Source: CAD feature listing. Evaluate the final solid. Frame: model axes, mm. A direction names the side the tool comes from. Coordinates: 2 decimals unless noted, no trailing zeros. Order: outer loops, then holes, each group sorted by start corner. A loop starts at its lowest first (then second) coordinate and runs counter-clockwise, first axis right, second up.
```python
from build123d import *

# Parameters (mm, degrees)
F0_W     = 46.8558967113
F0_H     = 64.1569495201
F1_DEPTH = 127
F2_R     = 23.3551916442
F2_W     = 46.8558967113
F2_H     = 64.1569495201
F2_R_2   = 20.2511661355
F3_DEPTH = 25.4


# Not quite as in the source:
# - a feature of the source that left no trace in its solid (it failed there, or was rolled back) is left out


with BuildPart() as f1:
    # F0 (on Top) → F1 (new body)
    with BuildSketch(Plane.XY):
        Rectangle(F0_W, F0_H)
    extrude(amount=F1_DEPTH)

    # F0 (on Top) + F2 (on face) → F3 (join)
    with BuildSketch(Plane.XY):
        Rectangle(F0_W, F0_H)
    with BuildSketch(Plane.XY):
        with BuildLine():
            Line((33.4399625558, -78.6570606891), (35.4419024774, -78.6570606891))
            Line((35.4419024774, -78.6570606891), (35.4419024774, 78.6570606891))
            ThreePointArc((35.4419024774, 78.6570606891), (0, 114.0989631665), (-35.4419024774, 78.6570606891))
            Line((-35.4419024774, 78.6570606891), (-35.4419024774, -78.6570606891))
            Line((-35.4419024774, -78.6570606891), (-33.4399625558, -78.6570606891))
            ThreePointArc((-33.4399625558, -78.6570606891), (0, -112.0970232449), (33.4399625558, -78.6570606891))
        make_face()
        with Locations((0, -78.6570606891)):
            Circle(F2_R, mode=Mode.SUBTRACT)
        Rectangle(F2_W, F2_H, mode=Mode.SUBTRACT)
        with Locations((0, 78.6570606891)):
            Circle(F2_R_2, mode=Mode.SUBTRACT)
    extrude(amount=F3_DEPTH)


solid = f1.part
```
1. Section query A-A on x = 0. Return loops of the section in (y, z), plus the area to 3 significant figures.
Findings:
outline: (-112.1, 0) - (-102.01, 0) - (-102.01, 25.4) - (-112.1, 25.4) - close; (-55.3, 0) - (58.41, 0) - (58.41, 25.4) - (32.08, 25.4) - (32.08, 127) - (-32.08, 127) - (-32.08, 25.4) - (-55.3, 25.4) - close; (98.91, 0) - (114.1, 0) - (114.1, 25.4) - (98.91, 25.4) - close
area: 10,000 mm2
2. Ray query, line 1 (Y direction, x = 0, z = 12); line 2 (Z direction, x = 14.5, y = 45); line 3 (Y direction, x = 12, z = 63.5). Return the intervals inside material, ascending.
Findings:
line 1: y = -112.1 to -102.01, -55.3 to 58.41, 98.91 to 114.1
line 2: z = 0 to 25.4
line 3: y = -32.08 to 32.08
3. Section query B-B on y = -84. Return loops of the section in (x, z), plus the area to 3 significant figures.
Findings:
outline: (-33.01, 0) - (-22.74, 0) - (-22.74, 25.4) - (-33.01, 25.4) - close; (22.74, 0) - (33.01, 0) - (33.01, 25.4) - (22.74, 25.4) - close
area: 522 mm2
4. Draft query along X for faces 1 (the face through (35.442, -1, 13)), 2 (the face through (-0.74, -112.09, 12.52)), 3 (the face through (-5.063, -101.457, 12.522)). Return one class per face: released by +X, released by -X, zero draft, split by the parting line, or undercut.
Findings:
face 1: released by +X
face 2: split by the parting line
face 3: undercut
5. Access query for faces 4 (the face through (23.428, 0, 75)), 5 (the face through (-23.428, 0, 75)), 6 (the face through (0, 32.078, 75)), 7 (the face through (0, -32.078, 75)). Directions: +Z, -Z, +X, -X, +Y, -Y. A direction counts if a zero-diameter tool reaches every point of the face in a straight line with its end or side. Return the directions, or none.
Findings:
face 4: +Z, +X, +Y, -Y
face 5: +Z, -X, +Y, -Y
face 6: +Z, +X, -X, +Y
face 7: +Z, +X, -X, -Y
6. Section query C-C on y = -9. Return loops of the section in (x, z).
Findings:
outline: (-35.44, 0) - (35.44, 0) - (35.44, 25.4) - (23.43, 25.4) - (23.43, 127) - (-23.43, 127) - (-23.43, 25.4) - (-35.44, 25.4) - close
7. Pin query (flat end, axial travel): P1, Ø0.6, axis at x = 35, z = 15.5, coming from the -Y side; P2, Ø8, axis at y = 13, z = 61, coming from the -X side; P3, Ø8, axis at x = 4.5, z = 45, coming from the -Y side. Return the tip coordinate at first contact, or that it passes through.
Findings:
P1: stops at y = -78.66
P2: stops at x = -23.43
P3: stops at y = -32.08
8. Section query D-D on z = 42.5. Return loops of the section in (x, y), plus the area to 3 significant figures.
Findings:
outline: (-23.43, -32.08) - (23.43, -32.08) - (23.43, 32.08) - (-23.43, 32.08) - close
area: 3,010 mm2
